Check sheet for the modelled part. Datum: model origin and axes. Units: mm. A direction names the side the tool comes from. Give positions to 0.01 mm unless a question says otherwise; leave off trailing zeros. Order: outer loops, then holes, each group sorted by start corner. A loop starts at its lowest first (then second) coordinate and runs counter-clockwise, first axis right, second up.
from build123d import *

# Parameters (mm, degrees)
EXTRUDE1_DEPTH = 8.382
FILLET1_R      = 6.35
FILLET2_R      = 3.81


with BuildPart() as part:
    # Sketch1 → Extrude1 (new body)
    with BuildSketch(Plane.XY):
        with BuildLine():
            Line((0, 0), (12.7, 31.75))
            Line((12.7, 31.75), (12.7, 44.45))
            Line((12.7, 44.45), (47.625, 47.625))
            ThreePointArc((47.625, 47.625), (42.899438593, 33.68617349), (44.45, 19.05))
            Line((44.45, 19.05), (50.8, 0))
            Line((50.8, 0), (0, 0))
        make_face()
    extrude(amount=EXTRUDE1_DEPTH)

    # Fillet1
    fillet1_edges = [part.edges().sort_by_distance(p)[0] for p in [
        (12.7, 31.75, 4.191),
        (12.7, 44.45, 4.191),
    ]]
    fillet(fillet1_edges, radius=FILLET1_R)

    # Fillet2
    fillet2_edges = [part.edges().sort_by_distance(p)[0] for p in [
        (0, 0, 4.191),
        (50.8, 0, 4.191),
    ]]
    fillet(fillet2_edges, radius=FILLET2_R)


solid = part.part
1) Section check C-C, the plane y = 6. Record the cut outline in (x, z), then the cut area to 3 significant figures.
Recorded:
outline: (2.4, 0) - (48.8, 0) - (48.8, 8.38) - (2.4, 8.38) - close
area: 389 mm2
2) Depth check by flat-ended pin: pin 1 Ø5 at (y, z) = (40, 6.5) entering from +X; pin 2 Ø1.7 at (y, z) = (37, 4.5) entering from -X; pin 3 Ø8 at (x, y) = (6.5, 41) entering from -Z. Enter the tip coordinate at first touch or a pass-through.
Recorded:
pin 1: stops at x = 45.09
pin 2: stops at x = 12.7
pin 3: passes through
3) Section check B-B, the plane x = 46.5. Record the cut outline in (y, z).
Recorded:
outline: (0.13, 0) - (12.9, 0) - (12.9, 8.38) - (0.13, 8.38) - close; (45.61, 0) - (47.52, 0) - (47.52, 8.38) - (45.61, 8.38) - close
4) Material ranges on L1, parallel to Y at x = 24.5, z = 5.5; L2, parallel to X at y = 37, z = 0.75; L3, parallel to Y at x = 26.5, z = 6.5, recorded low to high.
Recorded:
L1: y = 0 to 45.52
L2: x = 12.7 to 43.43
L3: y = 0 to 45.7
5) Set-up check for faces 1 (the face through (46.756, 12.131, 4.132)), 2 (the face through (2.44, 1.72, 4.25)), 3 (the face through (12.7, 36, 4)): record each of +Z, -Z, +X, -X, +Y, -Y from which the full face is reachable in a straight line by a thin tool's end or side.
Recorded:
face 1: +Z, -Z, +X
face 2: +Z, -Z, -X
face 3: +Z, -Z, -X, +Y
6) Draft check along Y on faces 4 (the face through (42.923, 33.892, 4.132)), 5 (the face through (7.097, 17.742, 4.132)), 6 (the face through (26, 19, 0)). Enter one of: +Y half, -Y half, draft (parallel to the pull), parting line (faces both ways), or undercut.
Recorded:
face 4: undercut
face 5: +Y half
face 6: draft
7) Section check D-D, the plane x = 17.5. Record the cut outline in (y, z).
Recorded:
outline: (0, 0) - (44.81, 0) - (44.81, 8.38) - (0, 8.38) - close
